```python
from build123d import *

# Parameters (mm, degrees)
F0_R     = 5.753175
F0_R_2   = 6
F0_R_3   = 5.998256
F1_DEPTH = 40
F3_DEPTH = 10


with BuildPart() as f1:
    # F0 (on Top) → F1 (new body)
    with BuildSketch(Plane.XY):
        with BuildLine():
            ThreePointArc((25, 22), (24.12132, 24.12132), (22, 25))
            Line((22, 25), (-22, 25))
            ThreePointArc((-22, 25), (-24.12132, 24.12132), (-25, 22))
            Line((-25, 22), (-25, -22))
            ThreePointArc((-25, -22), (-24.12132, -24.12132), (-22, -25))
            Line((-22, -25), (22, -25))
            ThreePointArc((22, -25), (24.12132, -24.12132), (25, -22))
            Line((25, -22), (25, 22))
        make_face()
        with Locations((-15, -15)):
            Circle(F0_R, mode=Mode.SUBTRACT)
        with Locations((0, -15)):
            Circle(F0_R_2, mode=Mode.SUBTRACT)
        with Locations((15, -15)):
            Circle(F0_R_2, mode=Mode.SUBTRACT)
        with Locations((-15, 0)):
            Circle(F0_R, mode=Mode.SUBTRACT)
        with Locations((-15, 15)):
            Circle(F0_R_3, mode=Mode.SUBTRACT)
        Circle(F0_R_2, mode=Mode.SUBTRACT)
        with Locations((15, 0)):
            Circle(F0_R_2, mode=Mode.SUBTRACT)
        with Locations((0, 15)):
            Circle(F0_R_2, mode=Mode.SUBTRACT)
        with Locations((15, 15)):
            Circle(F0_R_3, mode=Mode.SUBTRACT)
    extrude(amount=F1_DEPTH)

    # F2 (on face) → F3 (join)
    with BuildSketch(Plane(origin=(0, 0, 0), x_dir=(1, 0, 0), z_dir=(0, 0, -1))):
        with BuildLine():
            ThreePointArc((25, 22), (24.12132, 24.12132), (22, 25))
            Line((22, 25), (-22, 25))
            ThreePointArc((-22, 25), (-24.12132, 24.12132), (-25, 22))
            Line((-25, 22), (-25, -22))
            ThreePointArc((-25, -22), (-24.12132, -24.12132), (-22, -25))
            Line((-22, -25), (22, -25))
            ThreePointArc((22, -25), (24.12132, -24.12132), (25, -22))
            Line((25, -22), (25, 22))
        make_face()
    extrude(amount=F3_DEPTH)


solid = f1.part
```
Geometry check sheet. Reference: the model listing, model coordinates, mm. A direction names the side the tool comes from. Give positions to 0.01 mm unless a question says otherwise; leave off trailing zeros. Order: outer loops, then holes, each group sorted by start corner. A loop starts at its lowest first (then second) coordinate and runs counter-clockwise, first axis right, second up.
1. Release check for a two-part mould opening along Y. For faces 1 (the face through (-24.1, -24.14, 15.35)), 2 (the face through (20.54, -2.3, 19.72)), 3 (the face through (0, 25, 15)) record: pulls with the +Y half, pulls with the -Y half, needs draft (parallel to the pull), parting line crosses it, or undercut.
2. Section check A-A, the plane z = 7. Give the number of separate pieces and of enclosed holes in the cut face, and give its area (3 significant figures).
3. Access from +Z, -Z, +X, -X, +Y, -Y to the whole of each face (thin tool, end or side, straight path). Record for faces 4 (the face through (-15, -15, 0)), 5 (the face through (25, 0, 15)).
4. Section check B-B, the plane x = 0. Enter the section's corners in (y, z).
5. Thickness scan on L1, parallel to Y at x = 0, z = 19; L2, parallel to Y at x = 2.5, z = 6; L3, parallel to X at y = 2.5, z = 24.5. Record the ranges inside material, lowest first.
6. Section check C-C, the plane y = 0. Enter the section's corners in (x, z), and give its area (3 significant figures).
7. Gauge pin test, flat end, axial feed: pin 1 Ø3.5 at (x, y) = (-13.5, 13.5) entering from +Z. Record the tip position at first contact, or that the pin passes through.
Values follow:
1. face 1: pulls with the -Y half
1. face 2: undercut
1. face 3: pulls with the +Y half
2. separate pieces: 1
2. enclosed holes: 9
2. area: 1,490 mm2
3. face 4: +Z
3. face 5: +Z, -Z, +X, +Y, -Y
4. outline: (-25, -10) - (25, -10) - (25, 40) - (21, 40) - (21, 0) - (9, 0) - (9, 40) - (6, 40) - (6, 0) - (-6, 0) - (-6, 40) - (-9, 40) - (-9, 0) - (-21, 0) - (-21, 40) - (-25, 40) - close
5. L1: y = -25 to -21, -9 to -6, 6 to 9, 21 to 25
5. L2: y = -25 to -20.45, -9.55 to -5.45, 5.45 to 9.55, 20.45 to 25
5. L3: x = -25 to -20.18, -9.82 to -5.45, 5.45 to 9.55, 20.45 to 25
6. outline: (-25, -10) - (25, -10) - (25, 40) - (21, 40) - (21, 0) - (9, 0) - (9, 40) - (6, 40) - (6, 0) - (-6, 0) - (-6, 40) - (-9.25, 40) - (-9.25, 0) - (-20.75, 0) - (-20.75, 40) - (-25, 40) - close
6. area: 1,080 mm2
7. pin 1: stops at z = 0
